Part model, mm, in its own coordinate system. Coordinates: 2 decimals unless noted, no trailing zeros. Write each loop counter-clockwise with the first axis right and the second up, starting at its lowest first coordinate (ties: lowest second). Pieces come first, ordered by that corner, then holes. Notation, with made-up numbers: (-5, 53) -> (53, 53) arc R14 ccw to (53, 77) -> close; hole circle Ø10 at (-21.75, -27). An arc over 180 degrees is marked (long way). Write item = value, one per line.
Autodesk Inventor part; units mm, degrees
ref_plane "YZ Plane" through (0, 0, 0) normal (1, 0, 0) x (0, 1, 0)
ref_plane "XZ Plane" through (0, 0, 0) normal (0, 1, 0) x (-1, 0, 0)
ref_plane "XY Plane" through (0, 0, 0) normal (0, 0, 1) x (1, 0, 0)
sketch "Sketch1" plane through (0, 0, 0) normal (0, 0, 1) x (1, 0, 0)
  circle A0 centre (0, 0) radius 15.875
  arc A1 (-30.226, 44.7179) -> (30.226, 44.7179) centre (0, 0) ccw
  circle A2 centre (0, 0) radius 22.5683 construction
  circle A3 centre (0, 0) radius 34.925 construction
  circle A4 centre (0, 34.925) radius 3.175
  line L0 (0, 41.275) -> (0, 0) construction
  line L1 (-19.05, 65.7616) -> (-19.05, 95.25)
  line L2 (-6.35, 107.95) -> (6.35, 107.95)
  line L3 (19.05, 95.25) -> (19.05, 65.7616)
  line L4 (0, 0) -> (0, 107.95) construction
  circle A5 centre (0, 88.9) radius 3.175
  circle A6 centre (-30.2459, -17.4625) radius 3.175
  circle A7 centre (30.2459, -17.4625) radius 3.175
  arc A8 (-30.226, 44.7179) -> (-19.05, 65.7616) centre (-44.45, 65.7616) ccw
  arc A9 (19.05, 65.7616) -> (30.226, 44.7179) centre (44.45, 65.7616) ccw
  arc A10 (-6.35, 107.95) -> (-19.05, 95.25) centre (-6.35, 95.25) ccw
  arc A11 (19.05, 95.25) -> (6.35, 107.95) centre (6.35, 95.25) ccw
  point P0 (-19.05, 107.95)
  point P1 (19.05, 107.95)
  point P2 (19.05, 50.5015)
  point P3 (-19.05, 50.5015)
  dimension "d0" = 107.95
  dimension "d2" = 31.75
  dimension "d6" = 6.35
  dimension "d14" = 19.05
  dimension "d15" = 6.35
  dimension "d16" = 19.05
  dimension "d18" = 88.9
  dimension "d22" = 360
  dimension "d26" = 25.4
  dimension "d29" = 12.7
  dimension "d30" = 19.05
extrude "Extrusion1" add sketch "Sketch1" along normal blind 2.54
properties part number "door_clamp"
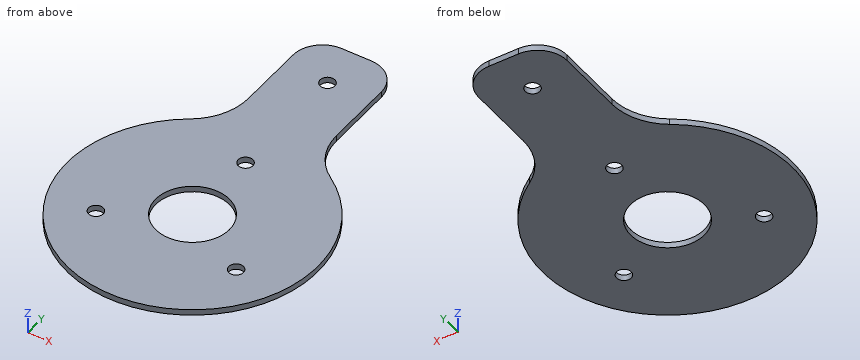
Q1. Saw through at D-D on y = 88.9. Give the cut face in (x, z) (3 decimals).
Model answer:
outline = (-19.05, 0) -> (-3.175, 0) -> (-3.175, 2.54) -> (-19.05, 2.54) -> close; (3.175, 0) -> (19.05, 0) -> (19.05, 2.54) -> (3.175, 2.54) -> close
Q2. Saw through at C-C on z = 1. Count the separate pieces of the cut face and the enclosed holes in it, and give its area (3 significant figures).
Model answer:
separate_pieces = 1
enclosed_holes = 5
area = 10,300 mm²
Q3. Probe line 1 (Y direction, x = -0.5, z = 1.15); line 2 (Y direction, x = 1, z = 1.7); line 3 (X direction, y = 64.5, z = 1.85). List the from-to ranges inside material, lowest first. Write a range as from..to.
Model answer:
line_1 = -53.97..-15.87, 15.87..31.79, 38.06..85.76, 92.04..107.95
line_2 = -53.97..-15.84, 15.84..31.91, 37.94..85.89, 91.91..107.95
line_3 = -19.08..19.08
Q4. Pin check, flat tips, straight feed: pin 1 (4 mm diameter, centred on x = 0, y = 34.925, fed in from +Z); pin 2 (1 mm diameter, centred on y = -24.5, z = 0.5, fed in from -X); pin 3 (0.8 mm diameter, centred on y = 79.5, z = 0.5, fed in from +X); pin 4 (8.5 mm diameter, centred on x = -30.25, y = -17.46, fed in from +Z). Stop position of each tip, or through.
Model answer:
pin_1 = through
pin_2 = -48.35
pin_3 = 19.05
pin_4 = 2.54
Q5. Saw through at A-A on y = 0. Give the cut face in (x, z) (3 decimals), and give its area (3 significant figures).
Model answer:
outline = (-53.975, 0) -> (-15.875, 0) -> (-15.875, 2.54) -> (-53.975, 2.54) -> close; (15.875, 0) -> (53.975, 0) -> (53.975, 2.54) -> (15.875, 2.54) -> close
area = 194 mm²
Q6. Saw through at B-B on x = 0. Give the cut face in (y, z) (3 decimals).
Model answer:
outline = (-53.975, 0) -> (-15.875, 0) -> (-15.875, 2.54) -> (-53.975, 2.54) -> close; (15.875, 0) -> (31.75, 0) -> (31.75, 2.54) -> (15.875, 2.54) -> close; (38.1, 0) -> (85.725, 0) -> (85.725, 2.54) -> (38.1, 2.54) -> close; (92.075, 0) -> (107.95, 0) -> (107.95, 2.54) -> (92.075, 2.54) -> close
